```python
from build123d import *

# Parameters (mm, degrees)
SKETCH2_R           = 3.81
BOSS_EXTRUDE1_DEPTH = 10.16
SKETCH3_R           = 2.54
BOSS_EXTRUDE2_DEPTH = 5.08
BOSS_EXTRUDE3_START = 5.08
SKETCH4_R           = 2.54
BOSS_EXTRUDE3_DEPTH = 5.08
SKETCH5_R           = 3.81
BOSS_EXTRUDE4_DEPTH = 5.08
SKETCH6_R           = 2.54
BOSS_EXTRUDE5_DEPTH = 5.08


with BuildPart() as part:
    # Sketch2 → Boss-Extrude1 (new body)
    with BuildSketch(Plane.XY):
        Circle(SKETCH2_R)
    extrude(amount=BOSS_EXTRUDE1_DEPTH)

    # Sketch3 → Boss-Extrude2 (add)
    with BuildSketch(Plane.XY.offset(10.16)):
        Circle(SKETCH3_R)
    extrude(amount=BOSS_EXTRUDE2_DEPTH)

    # Sketch4 → Boss-Extrude3 (add)
    with BuildSketch(Plane(origin=(0, 0, 0), x_dir=(-1, 0, 0), z_dir=(0, 0, -1)).offset(BOSS_EXTRUDE3_START)):
        with Locations(Location((0, 0, 0), (0, 0, 180))):
            Circle(SKETCH4_R)
    extrude(amount=-BOSS_EXTRUDE3_DEPTH)

    # Sketch5 → Boss-Extrude4 (add)
    with BuildSketch(Plane(origin=(0, 0, 0), x_dir=(1, 0, 0), z_dir=(0, 1, 0))):
        with Locations((0, -5.08)):
            Circle(SKETCH5_R)
    extrude(amount=BOSS_EXTRUDE4_DEPTH)

    # Sketch6 → Boss-Extrude5 (add)
    with BuildSketch(Plane(origin=(0, 5.08, 0), x_dir=(1, 0, 0), z_dir=(0, 1, 0))):
        with Locations(Location((0, -5.08, 0), (0, 0, 270))):
            Circle(SKETCH6_R)
    extrude(amount=BOSS_EXTRUDE5_DEPTH)


solid = part.part
```
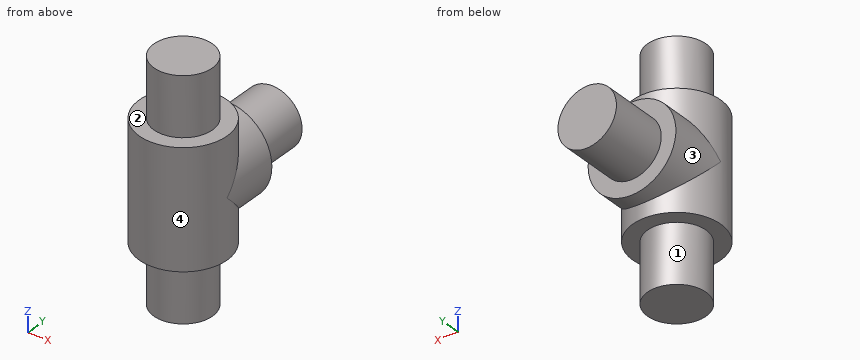
Read the model definition and answer for the solid it produces. Units are mm, in the model's axes. Face numbers are marked on the shaded views. A direction names the side the tool comes from. Round coordinates to 2 decimals unless told otherwise and drop trailing zeros. Write each loop counter-clockwise with the first axis right and the second up, starting at its lowest first coordinate (ties: lowest second). Pieces come first, ordered by that corner, then holes. Notation, with made-up numbers: (-8, 73) -> (34, 73) arc R4 ccw to (34, 77) -> close; hole circle Ø7 at (-29, -30.5). An arc over 180 degrees is marked (long way). Answer in a Markdown table with one row per item. Add a question column.
1) Find section A-A, the plane x = 0. Determine the outline of the cut face in (y, z), and give its area (3 significant figures).
2) Consider line 1 (Z direction, x = 3, y = 1.25); line 2 (X direction, y = 2.75, z = 9); line 3 (Z direction, x = -2, y = 7.75). Determine where each line is inside the solid, lowest interval first.
3) Given P1, Ø3, axis at x = -2.5, z = 1, coming from the +Y side; P2, Ø2, axis at x = 2.5, y = 7.5, coming from the -Z side, each flat-ended and moving along its own axis, determine where each tip first touches the part or whether it passes through.
4) Find section C-C, the plane y = 0.25. Determine the outline of the cut face in (x, z).
5) Find section D-D, the plane x = -2.75. Determine the outline of the cut face in (y, z).
6) Find section B-B, the plane z = 5.08. Determine the outline of the cut face in (x, y).
7) Which of the six approach directions +Z, -Z, +X, -X, +Y, -Y give full straight-line access (tool end or side, diameter ignored) to the marked faces 1, 2, 3 and 4?
Findings below:
| question | item | result |
|---|---|---|
| 1 | outline | (-3.81, 0) -> (-2.54, 0) -> (-2.54, -5.08) -> (2.54, -5.08) -> (2.54, 0) -> (3.81, 0) -> (3.81, 1.27) -> (5.08, 1.27) -> (5.08, 2.54) -> (10.16, 2.54) -> (10.16, 7.62) -> (5.08, 7.62) -> (5.08, 8.89) -> (3.81, 8.89) -> (3.81, 10.16) -> (2.54, 10.16) -> (2.54, 15.24) -> (-2.54, 15.24) -> (-2.54, 10.16) -> (-3.81, 10.16) -> close |
| 1 | area | 165 mm² |
| 2 | line 1 | 0 to 10.16 |
| 2 | line 2 | -2.64 to 2.64 |
| 2 | line 3 | 3.51 to 6.65 |
| 3 | P1 | y = 5.08 |
| 3 | P2 | z = 3.03 |
| 4 | outline | (-3.8, 0) -> (-2.53, 0) -> (-2.53, -5.08) -> (2.53, -5.08) -> (2.53, 0) -> (3.8, 0) -> (3.8, 4.83) arc R3.81 ccw to (3.8, 5.33) -> (3.8, 10.16) -> (2.53, 10.16) -> (2.53, 15.24) -> (-2.53, 15.24) -> (-2.53, 10.16) -> (-3.8, 10.16) -> (-3.8, 5.33) arc R3.81 ccw to (-3.8, 4.83) -> close |
| 5 | outline | (-2.64, 0) -> (2.64, 0) -> (2.64, 2.44) -> (5.08, 2.44) -> (5.08, 7.72) -> (2.64, 7.72) -> (2.64, 10.16) -> (-2.64, 10.16) -> close |
| 6 | outline | (-3.81, 0) arc R3.81 ccw to (3.81, 0) -> (3.81, 5.08) -> (2.54, 5.08) -> (2.54, 10.16) -> (-2.54, 10.16) -> (-2.54, 5.08) -> (-3.81, 5.08) -> close |
| 7 | face 1 | -Z |
| 7 | face 2 | +Z |
| 7 | face 3 | +Y |
| 7 | face 4 | none |
